Part model, mm, in its own coordinate system. Give positions to 0.01 mm unless a question says otherwise; leave off trailing zeros. Loops run counter-clockwise (first coordinate to the right, second up) from the corner with the lowest first, then second, coordinate; pieces in that order, holes last. Notation, with made-up numbers: (-11.5, 53.25) -> (1.5, 53.25) arc R23 cw to (1.5, 62.25) -> close; hole circle Ø9 at (83, 62). An arc over 180 degrees is marked (long way). Write item = value, one per line.
from build123d import *

# Parameters (mm, degrees)
SKETCH_1_W          = 85
SKETCH_1_H          = 55
EXTRUDE_1_DEPTH     = 0.5
CUT_EXTRUDE_1_REACH = 52.624
FILLET_1_R          = 2


with BuildPart() as part:
    # 草图1 → 凸台-拉伸1 (new body)
    with BuildSketch(Plane.XY):
        Rectangle(SKETCH_1_W, SKETCH_1_H)
    extrude(amount=EXTRUDE_1_DEPTH)

    # 草图2 → 切除-拉伸1 (cut, up to next)
    with BuildSketch(Plane.XY.offset(0.5), mode=Mode.PRIVATE) as cut_extrude_1_sk1:
        with BuildLine():
            Line((-37.5, 24.5), (39, 24.5))
            ThreePointArc((39, 24.5), (39.707106781, 24.207106781), (40, 23.5))
            Line((40, 23.5), (40, -16.5))
            ThreePointArc((40, -16.5), (39.707106781, -17.207106781), (39, -17.5))
            Line((39, -17.5), (-37.5, -17.5))
            ThreePointArc((-37.5, -17.5), (-38.207106781, -17.207106781), (-38.5, -16.5))
            Line((-38.5, -16.5), (-38.5, 23.5))
            ThreePointArc((-38.5, 23.5), (-38.207106781, 24.207106781), (-37.5, 24.5))
        make_face()
    cut_extrude_1_tool1 = extrude(cut_extrude_1_sk1.sketch, amount=-CUT_EXTRUDE_1_REACH, mode=Mode.PRIVATE) & part.part
    add(cut_extrude_1_tool1.solids().sort_by_distance((0.75, 3.5, 0.5))[0], mode=Mode.SUBTRACT)

    # 圆角1
    fillet_1_edges = [part.edges().sort_by_distance(p)[0] for p in [
        (42.5, -27.5, 0.25),
        (-42.5, -27.5, 0.25),
        (-42.5, 27.5, 0.25),
        (42.5, 27.5, 0.25),
    ]]
    fillet(fillet_1_edges, radius=FILLET_1_R)


solid = part.part
1) Slice it at C-C, the plane z = 0.15. List the corners of the cut face in (x, y).
Resolved:
outline = (-42.5, -25.5) arc R2 ccw to (-40.5, -27.5) -> (40.5, -27.5) arc R2 ccw to (42.5, -25.5) -> (42.5, 25.5) arc R2 ccw to (40.5, 27.5) -> (-40.5, 27.5) arc R2 ccw to (-42.5, 25.5) -> close; hole (-38.5, -16.5) arc R1 ccw to (-37.5, -17.5) -> (39, -17.5) arc R1 ccw to (40, -16.5) -> (40, 23.5) arc R1 ccw to (39, 24.5) -> (-37.5, 24.5) arc R1 ccw to (-38.5, 23.5) -> close
2) Slice it at B-B, the plane y = 6. List the corners of the cut face in (x, z).
Resolved:
outline = (-42.5, 0) -> (-38.5, 0) -> (-38.5, 0.5) -> (-42.5, 0.5) -> close; (40, 0) -> (42.5, 0) -> (42.5, 0.5) -> (40, 0.5) -> close
3) Drill centre lines: line 1 along X through (y, z) = (9.5, 0.25); line 2 along Y through (x, z) = (-32.5, 0.45). Where is each one in solid material? Low to high. Write a range as [from, to].
Resolved:
line_1 = [-42.5, -38.5], [40, 42.5]
line_2 = [-27.5, -17.5], [24.5, 27.5]
4) Slice it at A-A, the plane x = 24. List the corners of the cut face in (y, z), and give its area (3 significant figures).
Resolved:
outline = (-27.5, 0) -> (-17.5, 0) -> (-17.5, 0.5) -> (-27.5, 0.5) -> close; (24.5, 0) -> (27.5, 0) -> (27.5, 0.5) -> (24.5, 0.5) -> close
area = 6.50 mm²
